Design review of the part built by this model. Coordinates are the model's own, in mm. Face numbers are marked on the shaded views. Coordinates: 2 decimals unless noted, no trailing zeros. Loops run counter-clockwise (first coordinate to the right, second up) from the corner with the lowest first, then second, coordinate; pieces in that order, holes last. Notation, with made-up numbers: (2, 78.25) - (15, 78.25) arc R22 cw to (15, 101.25) - close; hole circle Ø9 at (8.5, -36.75). An arc over 180 degrees is marked (long way). Answer in a Markdown table with one row per item. Add a question column.
(1) We need section D-D, the plane z = 0. Write out the cut boundary in (x, y) (3 decimals).
(2) We need section B-B, the plane z = 60. Write out the cut boundary in (x, y).
(3) The part is to be moulded in two halves that separate along X. For the marked faces 1, 2 and 3, say which applies: released by +X, released by -X, zero draft, split by the parting line, or undercut.
(4) We need section A-A, the plane y = 114. Write out the cut boundary in (x, z) (3 decimals).
(5) To check wall thickness, follow L1, parallel to X at y = 6.25, z = -60; L2, parallel to Z at x = 0, y = 58 (3 decimals). State the ranges of each line that lie inside material, in increasing order. Write a range as [from, to].
(6) Clearance check with flat-ended pins moving along their axes: pin 1 (1.8 mm diameter, centred on y = 109.5, z = -20, fed in from +X); pin 2 (1.2 mm diameter, centred on x = 0.5, z = -21, fed in from +Y); pin 3 (13 mm diameter, centred on x = -60, z = -60, fed in from -Y); pin 4 (4 mm diameter, centred on y = 125.5, z = 20, fed in from +X). State where each tip first meets the part, or that it passes through.
(7) We need section C-C, the plane x = 60. Write out the cut boundary in (y, z).
Autodesk Inventor part; units mm, degrees
ref_plane "YZ Plane" through (0, 0, 0) normal (1, 0, 0) x (0, 1, 0)
ref_plane "XZ Plane" through (0, 0, 0) normal (0, 1, 0) x (-1, 0, 0)
sketch "Sketch1" plane through (0, 0, 0) normal (0, 1, 0) x (-1, 0, 0)
  line L0 (75, 75) -> (-75, 75)
  line L1 (-75, 75) -> (-75, -75)
  line L2 (-75, -75) -> (75, -75)
  line L3 (75, -75) -> (75, 75)
  line L4 (75, 75) -> (-75, -75) construction
  line L5 (-75, 75) -> (75, -75) construction
  point P0 (0, 0)
  dimension "d6" = 150
  dimension "d7" = 150
extrude "Extrusion4" add sketch "Sketch1" along normal blind 10
sketch "Sketch4" plane through (0, 10, 0) normal (0, 1, 0) x (1, 0, 0)
  line L0 (75, 75) -> (-75, 75)
  line L1 (0, 0) -> (-75, 75) construction
  circle A0 centre (-60, 60) radius 5
  line L2 (-75, 75) -> (-75, -75)
  line L3 (0, 75) -> (0, -75) construction
  line L4 (-75, -75) -> (75, -75)
  line L5 (-75, 0) -> (75, 0) construction
  circle A1 centre (60, 60) radius 5
  circle A2 centre (-60, -60) radius 5
  circle A3 centre (60, -60) radius 5
  dimension "d10" = 10
  dimension "d11" = 15
  dimension "d12" = 15
extrude "Extrusion5" cut sketch "Sketch4" against normal through all
sketch "Sketch5" plane through (0, 10, 0) normal (0, 1, 0) x (1, 0, 0)
  circle A0 centre (0, 0) radius 22.5
  circle A1 centre (0, 0) radius 19.005
  dimension "d15" = 45
  dimension "d18" = 38.01
extrude "Extrusion6" add sketch "Sketch5" along normal blind 139
fillet "Fillet1" radius 5 1 edges at (-22.5, 10, 0)
ref_plane "Work Plane1" through (0, 10, 22.5) normal (0, 0, 1) x (1, 0, 0)
sketch "Sketch6" plane through (0, 10, 22.5) normal (0, 0, 1) x (1, 0, 0)
  line L0 (-5, 214) -> (5, 214)
  line L1 (5, 214) -> (5, 64)
  line L2 (5, 64) -> (-5, 64)
  line L3 (-5, 64) -> (-5, 214)
  line L4 (-19.005, 139) -> (19.005, 139)
  line L5 (-5, 214) -> (5, 64) construction
  line L6 (5, 214) -> (-5, 64) construction
  point P0 (0, -10)
  point P1 (0, 139)
  point P2 (5, 139)
  point P3 (-5, 139)
  dimension "d20" = 10
  dimension "d21" = 150
extrude "Extrusion7" cut sketch "Sketch6" against normal through all contours L4 L1 L2 L3
properties part number "Motor_beam_connection"
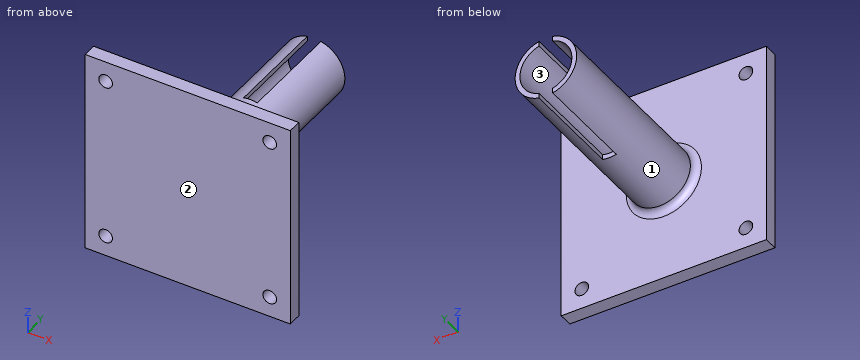
Responses:
| question | item | result |
|---|---|---|
| 1 | outline | (-75, 0) - (75, 0) - (75, 10) - (27.5, 10) arc R5 cw to (22.5, 15) - (22.5, 149) - (19.005, 149) - (19.005, 10) - (-19.005, 10) - (-19.005, 149) - (-22.5, 149) - (-22.5, 15) arc R5 cw to (-27.5, 10) - (-75, 10) - close |
| 2 | outline | (-75, 0) - (-65, 0) - (-65, 10) - (-75, 10) - close; (-55, 0) - (55, 0) - (55, 10) - (-55, 10) - close; (65, 0) - (75, 0) - (75, 10) - (65, 10) - close |
| 3 | face 1 | split by the parting line |
| 3 | face 2 | zero draft |
| 3 | face 3 | undercut |
| 4 | outline | (-5, -21.937) - (-5, -18.335) arc R19.005 cw to (-5, 18.335) - (-5, 21.937) arc R22.5 ccw to start; (5, -21.937) arc R22.5 ccw to (5, 21.937) - (5, 18.335) arc R19.005 cw to (5, -18.335) - close |
| 5 | L1 | x = [-75, -65], [-55, 55], [65, 75] |
| 5 | L2 | z = [-22.5, -19.005], [19.005, 22.5] |
| 6 | pin 1 | stops at x = 11.89 |
| 6 | pin 2 | stops at y = 74 |
| 6 | pin 3 | stops at y = 0 |
| 6 | pin 4 | stops at x = 13.5 |
| 7 | outline | (0, -75) - (10, -75) - (10, -65) - (0, -65) - close; (0, -55) - (10, -55) - (10, 55) - (0, 55) - close; (0, 65) - (10, 65) - (10, 75) - (0, 75) - close |
